```python
from build123d import *

# Parameters (mm, degrees)
SKETCH1_W                = 650
SKETCH1_H                = 650
BOSS_EXTRUDE1_DEPTH      = 8
BOSS_EXTRUDE2_DEPTH      = 650
CUT_EXTRUDE2_DEPTH       = 921.277302922
CUT_EXTRUDE2_DEPTH_BACK  = 921.277302922
SKETCH4_R                = 11
CUT_EXTRUDE1_DEPTH       = 920.932062709
CUT_EXTRUDE1_DEPTH_BACK  = 920.932062709
SKETCH2_R                = 210
CUT_EXTRUDE3_DEPTH       = 921.277302998
CUT_EXTRUDE3_DEPTH_BACK  = 110
CUT_EXTRUDE4_DEPTH       = 110
CUT_EXTRUDE5_DEPTH       = 920.932062713
CUT_EXTRUDE5_DEPTH_BACK  = 920.932062713
SKETCH7_OUTSIDE_W        = 836.056
SKETCH7_OUTSIDE_H        = 836.056
BOSS_EXTRUDE3_DEPTH      = 160.08
BOSS_EXTRUDE4_DEPTH      = 160.08
SKETCH21_W               = 10
SKETCH21_H               = 4.3
CUT_EXTRUDE10_DEPTH      = 680.197320372
SKETCH22_W               = 10
SKETCH22_H               = 4.3
CUT_EXTRUDE11_DEPTH      = 278.189465889
BOSS_EXTRUDE5_DEPTH      = 60
CUT_EXTRUDE6_DEPTH       = 679.914574891
CUT_EXTRUDE6_DEPTH_BACK  = 679.914574891
SKETCH12_R               = 210
CUT_EXTRUDE14_DEPTH      = 11
SKETCH27_R               = 2.2
SKETCH27_R_2             = 2.75
CUT_EXTRUDE15_DEPTH      = 11
SKETCH28_R               = 2.75
SKETCH28_R_2             = 2.2
CUT_EXTRUDE16_DEPTH      = 11
SKETCH29_W               = 20
SKETCH29_H               = 20
CUT_EXTRUDE17_DEPTH      = 10
CUT_EXTRUDE18_DEPTH      = 679.914574891
CUT_EXTRUDE18_DEPTH_BACK = 679.914574891
SKETCH30_W               = 95
SKETCH30_H               = 195
CUT_EXTRUDE19_DEPTH      = 679.914574891
CUT_EXTRUDE19_DEPTH_BACK = 679.914574891
SKETCH31_W               = 100
SKETCH31_H               = 75
SKETCH32_W               = 20.1
SKETCH32_H               = 20.1
CUT_EXTRUDE20_DEPTH      = 10
SKETCH33_R               = 2.15
CUT_EXTRUDE21_DEPTH      = 10
CHAMFER1_SIZE            = 1


with BuildPart() as part:
    # Sketch1 → Boss-Extrude1 (new body)
    with BuildSketch(Plane(origin=(0, 0, 0), x_dir=(1, 0, 0), z_dir=(0, 1, 0))):
        with Locations((325, 325)):
            Rectangle(SKETCH1_W, SKETCH1_H)
    extrude(amount=BOSS_EXTRUDE1_DEPTH)

    # Sketch3 → Boss-Extrude2 (add)
    with BuildSketch(Plane.XY):
        Polygon((300, 43.707142143), (350, 43.707142143), (385, 8), (265, 8), align=None)
    extrude(amount=-BOSS_EXTRUDE2_DEPTH)

    # Sketch4 → Cut-Extrude2 (cut, two sides: drawn at the far end of the back side and taken through both)
    with BuildSketch(Plane.XY.offset(-CUT_EXTRUDE2_DEPTH_BACK)):
        with Locations((325, 22)):
            Circle(SKETCH4_R)
    extrude(amount=CUT_EXTRUDE2_DEPTH + CUT_EXTRUDE2_DEPTH_BACK, mode=Mode.SUBTRACT)

    # Sketch2 → Cut-Extrude1 (cut, two sides: drawn at the far end of the back side and taken through both)
    with BuildSketch(Plane(origin=(0, 8, 0), x_dir=(1, 0, 0), z_dir=(0, 1, 0)).offset(-CUT_EXTRUDE1_DEPTH_BACK)):
        with Locations(Location((325, 325, 0), (0, 0, 270))):
            Circle(SKETCH2_R)
    extrude(amount=CUT_EXTRUDE1_DEPTH + CUT_EXTRUDE1_DEPTH_BACK, mode=Mode.SUBTRACT)

    # Sketch5 → Cut-Extrude3 (cut, two sides: drawn at the far end of the back side and taken through both)
    with BuildSketch(Plane.XY.offset(-CUT_EXTRUDE3_DEPTH_BACK)):
        Polygon((300, 43.707142143), (350, 43.707142143), (365.396078824, 28), (350, 28), (350, 8), (300, 8), (300, 28), (284.603921176, 28), align=None)
    extrude(amount=CUT_EXTRUDE3_DEPTH + CUT_EXTRUDE3_DEPTH_BACK, mode=Mode.SUBTRACT)

    # Sketch6 → Cut-Extrude4 (cut)
    with BuildSketch(Plane(origin=(0, 0, -650), x_dir=(-1, 0, 0), z_dir=(0, 0, -1))):
        Polygon((-350, 43.707142143), (-300, 43.707142143), (-284.603921176, 28), (-300, 28), (-300, 8), (-350, 8), (-350, 28), (-365.396078824, 28), align=None)
    extrude(amount=-CUT_EXTRUDE4_DEPTH, mode=Mode.SUBTRACT)

    # Sketch7 outside → Cut-Extrude5 (cut, two sides: drawn at the far end of the back side and taken through both)
    with BuildSketch(Plane(origin=(0, 8, 0), x_dir=(1, 0, 0), z_dir=(0, 1, 0)).offset(-CUT_EXTRUDE5_DEPTH_BACK)):
        with Locations((325, 325)):
            Rectangle(SKETCH7_OUTSIDE_W, SKETCH7_OUTSIDE_H)
        Polygon((195, 455), (195, 489.924225025), (195, 650), (167.478198198, 686.544504505), (-70.838918919, 686.544504505), (-70.838918919, 472.462112512), (0, 455), (160.075774975, 455), align=None, mode=Mode.SUBTRACT)
    extrude(amount=CUT_EXTRUDE5_DEPTH + CUT_EXTRUDE5_DEPTH_BACK, mode=Mode.SUBTRACT)

    # Sketch8 → Boss-Extrude3 (add)
    with BuildSketch(Plane(origin=(0, 0, -650), x_dir=(-1, 0, 0), z_dir=(0, 0, -1))):
        Polygon((-195, 8), (-195, 28), (-185, 28), (-185, 17), (-175, 8), align=None)
    extrude(amount=-BOSS_EXTRUDE3_DEPTH)

    # Sketch10 → Boss-Extrude4 (add)
    with BuildSketch(Plane.ZY):
        Polygon((-455, 8), (-455, 28), (-465, 28), (-465, 17), (-475, 8), align=None)
    extrude(amount=-BOSS_EXTRUDE4_DEPTH)

    # Sketch21 → Cut-Extrude10 (cut, through all)
    with BuildSketch(Plane.ZY):
        with Locations((-460, 5)):
            Rectangle(SKETCH21_W, SKETCH21_H)
    extrude(amount=-CUT_EXTRUDE10_DEPTH, mode=Mode.SUBTRACT)

    # Sketch22 → Cut-Extrude11 (cut, through all)
    with BuildSketch(Plane(origin=(0, 0, -650), x_dir=(-1, 0, 0), z_dir=(0, 0, -1))):
        with Locations((-190, 5)):
            Rectangle(SKETCH22_W, SKETCH22_H)
    extrude(amount=-CUT_EXTRUDE11_DEPTH, mode=Mode.SUBTRACT)

    # Sketch23 → Boss-Extrude5 (add)
    with BuildSketch(Plane.XY.offset(-489.92)):
        Polygon((194.99464011, 8), (195, 28), (160.08, 28), (160.08, 8), align=None)
    extrude(amount=BOSS_EXTRUDE5_DEPTH)

    # Sketch12 → Cut-Extrude6 (cut, two sides: drawn at the far end of the back side and taken through both)
    with BuildSketch(Plane(origin=(0, 8, 0), x_dir=(1, 0, 0), z_dir=(0, 1, 0)).offset(-CUT_EXTRUDE6_DEPTH_BACK)):
        with Locations((325, 325)):
            Circle(SKETCH12_R)
    extrude(amount=CUT_EXTRUDE6_DEPTH + CUT_EXTRUDE6_DEPTH_BACK, mode=Mode.SUBTRACT)

    # Sketch26 → Cut-Extrude14 (cut)
    with BuildSketch(Plane(origin=(0, 28, 0), x_dir=(1, 0, 0), z_dir=(0, 1, 0))):
        Polygon((185, 489.92), (160.08, 489.92), (160.08, 465), align=None)
    extrude(amount=-CUT_EXTRUDE14_DEPTH, mode=Mode.SUBTRACT)

    # Sketch27 → Cut-Extrude15 (cut)
    with BuildSketch(Plane.ZY.offset(-185)):
        with Locations((-610, 23)):
            Circle(SKETCH27_R)
        with Locations((-560, 23)):
            Circle(SKETCH27_R_2)
        with Locations((-520, 23)):
            Circle(SKETCH27_R_2)
    extrude(amount=-CUT_EXTRUDE15_DEPTH, mode=Mode.SUBTRACT)

    # Sketch28 → Cut-Extrude16 (cut)
    with BuildSketch(Plane(origin=(0, 0, -465), x_dir=(-1, 0, 0), z_dir=(0, 0, -1))):
        with Locations((-120, 23)):
            Circle(SKETCH28_R)
        with Locations((-80, 23)):
            Circle(SKETCH28_R_2)
        with Locations((-40, 23)):
            Circle(SKETCH28_R_2)
    extrude(amount=-CUT_EXTRUDE16_DEPTH, mode=Mode.SUBTRACT)

    # Sketch29 → Cut-Extrude17 (cut)
    with BuildSketch(Plane(origin=(0, 8, 0), x_dir=(1, 0, 0), z_dir=(0, 1, 0))):
        with Locations((10, 640)):
            Rectangle(SKETCH29_W, SKETCH29_H)
    extrude(amount=-CUT_EXTRUDE17_DEPTH, mode=Mode.SUBTRACT)

    # Sketch30 → Cut-Extrude18 (cut, two sides: drawn at the far end of the back side and taken through both)
    with BuildSketch(Plane(origin=(0, 8, 0), x_dir=(1, 0, 0), z_dir=(0, 1, 0)).offset(-CUT_EXTRUDE18_DEPTH_BACK)):
        with Locations((47.5, 552.5)):
            Rectangle(SKETCH30_W, SKETCH30_H)
    extrude(amount=CUT_EXTRUDE18_DEPTH + CUT_EXTRUDE18_DEPTH_BACK, mode=Mode.SUBTRACT)

    # Sketch31 → Cut-Extrude19 (cut, two sides: drawn at the far end of the back side and taken through both)
    with BuildSketch(Plane(origin=(0, 8, 0), x_dir=(1, 0, 0), z_dir=(0, 1, 0)).offset(-CUT_EXTRUDE19_DEPTH_BACK)):
        with Locations((145, 612.5)):
            Rectangle(SKETCH31_W, SKETCH31_H)
    extrude(amount=CUT_EXTRUDE19_DEPTH + CUT_EXTRUDE19_DEPTH_BACK, mode=Mode.SUBTRACT)

    # Sketch32 → Cut-Extrude20 (cut)
    with BuildSketch(Plane(origin=(0, 8, 0), x_dir=(1, 0, 0), z_dir=(0, 1, 0))):
        with Locations((105.05, 564.95)):
            Rectangle(SKETCH32_W, SKETCH32_H)
    extrude(amount=-CUT_EXTRUDE20_DEPTH, mode=Mode.SUBTRACT)

    # Sketch33 → Cut-Extrude21 (cut)
    with BuildSketch(Plane(origin=(0, 8, 0), x_dir=(1, 0, 0), z_dir=(0, 1, 0))):
        with Locations(Location((105, 524.9, 0), (0, 0, 270))):
            Circle(SKETCH33_R)
        with Locations(Location((145.1, 565, 0), (0, 0, 270))):
            Circle(SKETCH33_R)
    extrude(amount=-CUT_EXTRUDE21_DEPTH, mode=Mode.SUBTRACT)

    # Chamfer1
    chamfer1_edges = [part.edges().sort_by_distance(p)[0] for p in [
        (105, 8, -527.05),
        (145.1, 8, -567.15),
    ]]
    chamfer(chamfer1_edges, length=CHAMFER1_SIZE)


solid = part.part
```
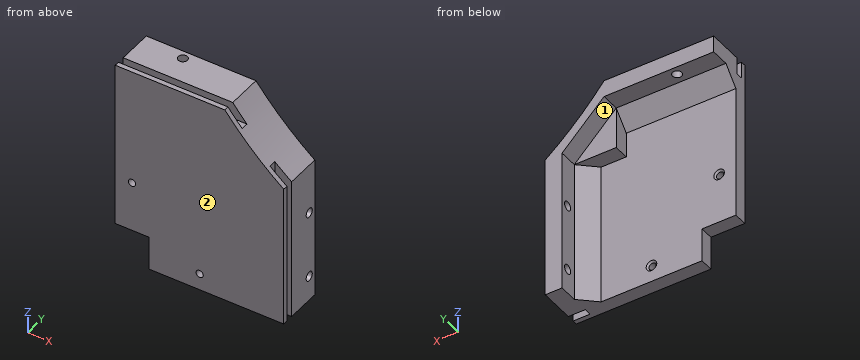
Input: part model. Units: mm. Frame: model coordinates. Face numbers are marked on the shaded views. A direction names the side the tool comes from. Coordinates: 2 decimals unless noted, no trailing zeros. Write each loop counter-clockwise with the first axis right and the second up, starting at its lowest first coordinate (ties: lowest second). Pieces come first, ordered by that corner, then holes. Notation, with made-up numbers: (11, 80.25) -> (49, 80.25) arc R9 ccw to (49, 84.25) -> close; hole circle Ø6 at (47, -34). An arc over 180 degrees is marked (long way). Answer as a JSON object with one key per item and string values.
1. First-contact query: P1, Ø8, axis at y = 20, z = -520.5, coming from the -X side; P2, Ø7, axis at y = 23, z = -520, coming from the -X side; P3, Ø5, axis at x = 105, z = -524.9, coming from the +Y side. Flat tips, straight axial feed; report the tip coordinate or a pass-through.
Result set:
{"P1": "stops at x = 183.89", "P2": "stops at x = 185", "P3": "stops at y = 7.35"}
2. Material intervals for line 1 (Y direction, x = 191.25, z = -520); line 2 (X direction, y = 4.75, z = -524.9); line 3 (Z direction, x = 145.1, y = 3.5), sorted ascending. Write a range as from..to.
Result set:
{"line 1": "y = 0..2.85, 7.15..20.25, 25.75..28", "line 2": "x = 95..102.85, 107.15..185", "line 3": "z = -575..-567.15, -562.85..-465"}
3. Section A-A on z = -560. Return the cut outline in (x, y).
Result set:
{"outline": "(115.1, 0) -> (195, 0) -> (195, 2.85) -> (185, 2.85) -> (185, 7.15) -> (195, 7.15) -> (195, 20.25) -> (185, 20.25) -> (185, 17) -> (175, 8) -> (115.1, 8) -> close; (185, 25.75) -> (195, 25.75) -> (195, 28) -> (185, 28) -> close"}
4. Section B-B on x = 145.1. Return the cut outline in (y, z), then the cut area to 3 significant figures.
Result set:
{"outline": "(0, -575) -> (8, -575) -> (8, -568.15) -> (7, -567.15) -> (0, -567.15) -> close; (0, -562.85) -> (7, -562.85) -> (8, -561.85) -> (8, -475) -> (17, -465) -> (28, -465) -> (28, -455) -> (7.15, -455) -> (7.15, -465) -> (2.85, -465) -> (2.85, -455) -> (0, -455) -> close", "area": "1,130 mm2"}
5. Section C-C on y = 23. Return the cut outline in (x, z), then the cut area to 3 significant figures.
Result set:
{"outline": "(95, -465) -> (117.25, -465) -> (117.25, -455) -> (95, -455) -> close; (122.75, -465) -> (160.08, -465) -> (185, -489.92) -> (185, -517.25) -> (195, -517.25) -> (195, -489.92) arc R210 cw to (160.08, -455) -> (122.75, -455) -> close; (185, -575) -> (195, -575) -> (195, -562.75) -> (185, -562.75) -> close; (185, -557.25) -> (195, -557.25) -> (195, -522.75) -> (185, -522.75) -> close", "area": "1,590 mm2"}
6. Access query for the marked faces 1 and 2. Directions: +Z, -Z, +X, -X, +Y, -Y. A direction counts if a zero-diameter tool reaches every point of the face in a straight line with its end or side. Return the directions, or none.
Result set:
{"face 1": "-Z, -X, +Y", "face 2": "+Z, -Z, +X, -X, -Y"}
7. Section D-D on z = -530.5. Return the cut outline in (x, y), then the cut area to 3 significant figures.
Result set:
{"outline": "(95, 0) -> (195, 0) -> (195, 2.85) -> (185, 2.85) -> (185, 7.15) -> (195, 7.15) -> (195, 28) -> (185, 28) -> (185, 17) -> (175, 8) -> (95, 8) -> close", "area": "1,000 mm2"}
